Part model, mm, in its own coordinate system. Give positions to 0.01 mm unless a question says otherwise; leave off trailing zeros. Write each loop counter-clockwise with the first axis right and the second up, starting at its lowest first coordinate (ties: lowest second). Pieces come first, ordered by that corner, then holes.
```python
from build123d import *

# Parameters (mm, degrees)
SKETCH_1_W          = 30
SKETCH_1_H          = 34
SKETCH_1_R          = 1.5
EXTRUDE_2_DEPTH     = 9.5
SKETCH_3_R          = 7.5
CUT_EXTRUDE_1_DEPTH = 40


with BuildPart() as part:
    # 草图1 → 凸台-拉伸2 (new body)
    with BuildSketch(Plane.XY):
        with Locations((-7.961038961, 0)):
            Rectangle(SKETCH_1_W, SKETCH_1_H)
        with Locations((1.038961039, 12)):
            Circle(SKETCH_1_R, mode=Mode.SUBTRACT)
        with Locations((-16.961038961, 12)):
            Circle(SKETCH_1_R, mode=Mode.SUBTRACT)
        with Locations((1.038961039, -12)):
            Circle(SKETCH_1_R, mode=Mode.SUBTRACT)
        with Locations((-16.961038961, -12)):
            Circle(SKETCH_1_R, mode=Mode.SUBTRACT)
    extrude(amount=EXTRUDE_2_DEPTH)

    # 草图3 → 切除-拉伸1 (cut)
    with BuildSketch(Plane.ZY.offset(22.961038961)):
        with Locations((9.5, 0)):
            Circle(SKETCH_3_R)
    extrude(amount=-CUT_EXTRUDE_1_DEPTH, mode=Mode.SUBTRACT)


solid = part.part
```
1) Saw through at C-C, the plane z = 4. Write the cut outline in (x, y).
Answers follow:
outline: (-22.96, -17) - (7.04, -17) - (7.04, -5.1) - (-22.96, -5.1) - close; (-22.96, 5.1) - (7.04, 5.1) - (7.04, 17) - (-22.96, 17) - close; hole circle Ø3 at (-16.96, -12); hole circle Ø3 at (-16.96, 12); hole circle Ø3 at (1.04, -12); hole circle Ø3 at (1.04, 12)
2) Saw through at A-A, the plane y = -12. Write the cut outline in (x, z), then the cut area to 3 significant figures.
Answers follow:
outline: (-22.96, 0) - (-18.46, 0) - (-18.46, 9.5) - (-22.96, 9.5) - close; (-15.46, 0) - (-0.46, 0) - (-0.46, 9.5) - (-15.46, 9.5) - close; (2.54, 0) - (7.04, 0) - (7.04, 9.5) - (2.54, 9.5) - close
area: 228 mm2
3) Saw through at D-D, the plane x = -5.25. Write the cut outline in (y, z).
Answers follow:
outline: (-17, 0) - (17, 0) - (17, 9.5) - (7.5, 9.5) arc R7.5 cw to (-7.5, 9.5) - (-17, 9.5) - close
4) Wall check: L1, parallel to Y at x = 2, z = 4; L2, parallel to Y at x = 3, z = 9.25; L3, parallel to X at y = -11, z = 7. Give the ranges that are in metal, low to high.
Answers follow:
L1: y = -17 to -13.15, -10.85 to -5.1, 5.1 to 10.85, 13.15 to 17
L2: y = -17 to -7.5, 7.5 to 17
L3: x = -22.96 to -18.08, -15.84 to -0.08, 2.16 to 7.04
5) Saw through at B-B, the plane z = 0.5. Write the cut outline in (x, y).
Answers follow:
outline: (-22.96, -17) - (7.04, -17) - (7.04, 17) - (-22.96, 17) - close; hole circle Ø3 at (-16.96, -12); hole circle Ø3 at (-16.96, 12); hole circle Ø3 at (1.04, -12); hole circle Ø3 at (1.04, 12)
6) Pin check, flat tips, straight feed: pin 1 Ø2.5 at (x, y) = (1.04, 12) entering from +Z; pin 2 Ø1.5 at (x, y) = (3, -13.5) entering from -Z. Stop position of each tip, or through.
Answers follow:
pin 1: passes through
pin 2: stops at z = 0
